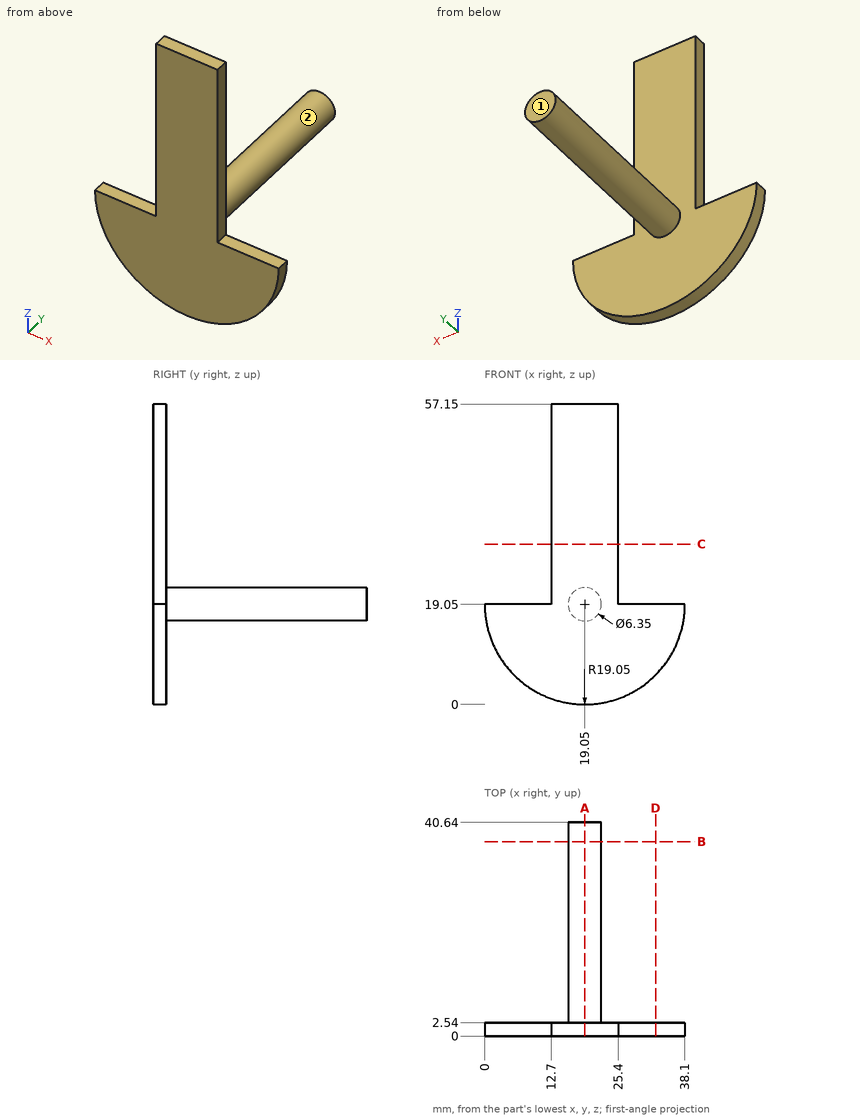
The figure shows three views and two pictorial views of one solid part (mm, origin at its lowest corner). Answer the questions. A direction names the side the tool comes from. Coordinates: 2 decimals unless noted, no trailing zeros. Loops run counter-clockwise (first coordinate to the right, second up) from the corner with the lowest first, then second, coordinate; pieces in that order, holes last. Notation, with made-up numbers: (-36, 9) - (1, 9) arc R18 ccw to (1, 31) - close; hole circle Ø4 at (77.5, 13.25). An arc over 180 degrees is marked (long way). Use a Markdown table: item, result. Add a question column.
1) Given pin 1 (1.3 mm diameter, centred on x = 7.5, y = 0.5, fed in from +Z); pin 2 (0.8 mm diameter, centred on y = 1, z = 32.5, fed in from +X); pin 3 (4 mm diameter, centred on x = 12.5, z = 38.5, fed in from +Y), each flat-ended and moving along its own axis, determine where each tip first touches the part or whether it passes through.
2) The part is cut by section D-D, the plane x = 32.5. Give the vertices of the cut face in (y, z), and give its area (3 significant figures).
3) The part is cut by section C-C, the plane z = 30.5. Give the vertices of the cut face in (x, y).
4) Find the intervals of material crossed by line 1 (Y direction, x = 16, z = 32); line 2 (X direction, y = 2, z = 52); line 3 (X direction, y = 37.5, z = 20.5), in increasing order.
5) The part is cut by section B-B, the plane y = 37. Give the vertices of the cut face in (x, z) (3 decimals), and give its area (3 significant figures).
6) The part is cut by section A-A, the plane x = 19.05. Give the vertices of the cut face in (y, z) (3 decimals), and give its area (3 significant figures).
7) For the marked faces 1 and 2, determine the directions among +Z, -Z, +X, -X, +Y, -Y from which every point of the face is accessible in a straight line to the end or side of a thin tool.
Here are the results:
| question | item | result |
|---|---|---|
| 1 | pin 1 | stops at z = 19.05 |
| 1 | pin 2 | stops at x = 25.4 |
| 1 | pin 3 | stops at y = 2.54 |
| 2 | outline | (0, 5.56) - (2.54, 5.56) - (2.54, 19.05) - (0, 19.05) - close |
| 2 | area | 34.3 mm^2 |
| 3 | outline | (12.7, 0) - (25.4, 0) - (25.4, 2.54) - (12.7, 2.54) - close |
| 4 | line 1 | y = 0 to 2.54 |
| 4 | line 2 | x = 12.7 to 25.4 |
| 4 | line 3 | x = 16.23 to 21.87 |
| 5 | outline | circle Ø6.35 at (19.05, 19.05) |
| 5 | area | 31.7 mm^2 |
| 6 | outline | (0, 0) - (2.54, 0) - (2.54, 15.875) - (40.64, 15.875) - (40.64, 22.225) - (2.54, 22.225) - (2.54, 57.15) - (0, 57.15) - close |
| 6 | area | 387 mm^2 |
| 7 | face 1 | +Z, -Z, +X, -X, +Y |
| 7 | face 2 | +Y |
